Here's the drawing with two shaded views (mm, measured from the low corner). I have some questions. Give positions to 0.01 mm unless a question says otherwise; leave off trailing zeros. Write each loop counter-clockwise with the first axis right and the second up, starting at its lowest first coordinate (ties: lowest second). Pieces come first, ordered by that corner, then holes. Notation, with made-up numbers: (35, 37) -> (64, 37) arc R21 ccw to (64, 64) -> close; hole circle Ø4 at (-14.75, 80.5). An arc over 180 degrees is marked (long way). One line per item, written item: value.
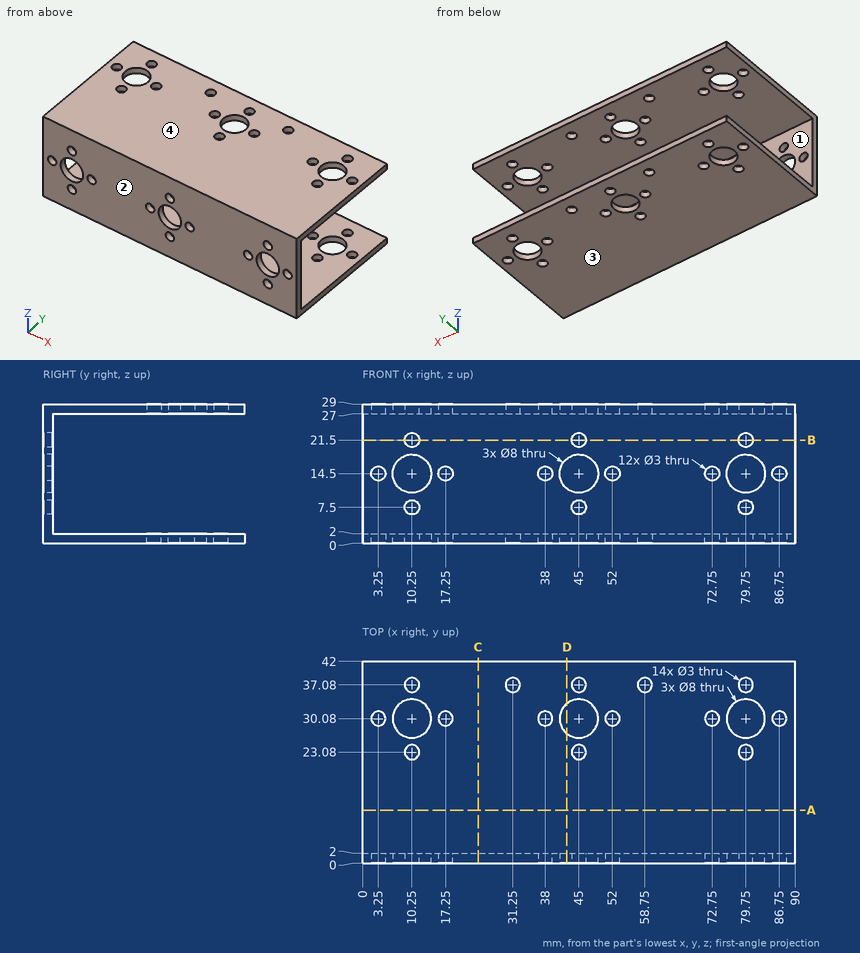
1) If we section it at C-C (x = 24): Write out the boundary of the cut face in (y, z), and give its area (3 significant figures).
Answer list:
outline: (0, 0) -> (42, 0) -> (42, 2) -> (2, 2) -> (2, 27) -> (42, 27) -> (42, 29) -> (0, 29) -> close
area: 218 mm^2
2) Will this pin go through, and if not, where does the flat tip stop? pin 1 (3.5 mm diameter, centred on x = 52, z = 14.5, fed in from +Y).
Answer list:
pin 1: stops at y = 2
3) If we section it at A-A (y = 11): Write out the boundary of the cut face in (x, z).
Answer list:
outline: (0, 0) -> (90, 0) -> (90, 2) -> (0, 2) -> close; (0, 27) -> (90, 27) -> (90, 29) -> (0, 29) -> close
4) I need wall thicknesses on L1, parallel to Y at x = 79.75, z = 27.8; L2, parallel to Z at x = 79.75, y = 0.45; L3, parallel to Y at x = 52, z = 0.5. Which ranges of each line are inside material? Lowest first, please.
Answer list:
L1: y = 0 to 21.58, 24.58 to 26.08, 34.08 to 35.58, 38.58 to 42
L2: z = 0 to 6, 9 to 10.5, 18.5 to 20, 23 to 29
L3: y = 0 to 28.58, 31.58 to 42
5) We'd pull the mould along Z, two halves only. Please class the marked faces 1, 2, 3 and 4: released by +Z, released by -Z, zero draft, split by the parting line, or undercut.
Answer list:
face 1: undercut
face 2: zero draft
face 3: released by -Z
face 4: released by +Z
6) If we section it at D-D (x = 42.5): Write out the boundary of the cut face in (y, z).
Answer list:
outline: (0, 0) -> (26.96, 0) -> (26.96, 2) -> (2, 2) -> (2, 11.38) -> (0, 11.38) -> close; (0, 17.62) -> (2, 17.62) -> (2, 27) -> (26.96, 27) -> (26.96, 29) -> (0, 29) -> close; (33.2, 0) -> (42, 0) -> (42, 2) -> (33.2, 2) -> close; (33.2, 27) -> (42, 27) -> (42, 29) -> (33.2, 29) -> close
7) If we section it at B-B (z = 21.5): Write out the boundary of the cut face in (x, y), and give its area (3 significant figures).
Answer list:
outline: (0, 0) -> (8.75, 0) -> (8.75, 2) -> (0, 2) -> close; (11.75, 0) -> (43.5, 0) -> (43.5, 2) -> (11.75, 2) -> close; (46.5, 0) -> (78.25, 0) -> (78.25, 2) -> (46.5, 2) -> close; (81.25, 0) -> (90, 0) -> (90, 2) -> (81.25, 2) -> close
area: 162 mm^2
